Verification items for the finished model (mm, model axes). A direction names the side the tool comes from. Coordinates: 2 decimals unless noted, no trailing zeros. Write each loop counter-clockwise with the first axis right and the second up, starting at its lowest first coordinate (ties: lowest second). Pieces come first, ordered by that corner, then holes. Notation, with made-up numbers: M 36,-20 L 59,-20 A21 cw 59,0 Z; hole C 33,88 d11. An arc over 180 degrees is marked long. Answer in a Markdown table with one row per item.
from build123d import *

# Parameters (mm, degrees)
SKETCH1_W           = 56.833752097
SKETCH1_H           = 5
BOSS_EXTRUDE1_DEPTH = 80
SKETCH2_W           = 18.416876048
SKETCH2_H           = 5
SKETCH2_W_2         = 18.416876049
BOSS_EXTRUDE2_DEPTH = 5
SKETCH3_W           = 20
SKETCH3_H           = 5
BOSS_EXTRUDE3_DEPTH = 5
CUT_EXTRUDE1_DEPTH  = 5
BOSS_EXTRUDE4_DEPTH = 5
SKETCH6_R           = 2.1
CUT_EXTRUDE2_DEPTH  = 5
SKETCH8_W           = 1.93349359
SKETCH8_H           = 7.9375
CUT_EXTRUDE3_DEPTH  = 5


with BuildPart() as part:
    # Sketch1 → Boss-Extrude1 (new body)
    with BuildSketch(Plane.XY):
        with Locations((-105.747769379, -71.943096951)):
            Rectangle(SKETCH1_W, SKETCH1_H)
    extrude(amount=BOSS_EXTRUDE1_DEPTH)

    # Sketch2 → Boss-Extrude2 (add)
    with BuildSketch(Plane(origin=(0, 0, 0), x_dir=(-1, 0, 0), z_dir=(0, 0, -1))):
        with Locations((86.539331354, -71.943096951)):
            Rectangle(SKETCH2_W, SKETCH2_H)
        with Locations((124.956207403, -71.943096951)):
            Rectangle(SKETCH2_W_2, SKETCH2_H)
    extrude(amount=BOSS_EXTRUDE2_DEPTH)

    # Sketch3 → Boss-Extrude3 (add)
    with BuildSketch(Plane.XY.offset(80)):
        with Locations((-105.747769378, -71.943096951)):
            Rectangle(SKETCH3_W, SKETCH3_H)
    extrude(amount=BOSS_EXTRUDE3_DEPTH)

    # Sketch4 → Cut-Extrude1 (cut)
    with BuildSketch(Plane.XZ.offset(74.443096951)):
        Polygon((-107.847769378, 0), (-107.847769378, 5), (-110.747769378, 5), (-110.747769378, 15), (-100.747769378, 15), (-100.747769378, 5), (-103.647769378, 5), (-103.647769378, 0), align=None)
    extrude(amount=-CUT_EXTRUDE1_DEPTH, mode=Mode.SUBTRACT)

    # Sketch5 → Boss-Extrude4 (add)
    with BuildSketch(Plane.XZ.offset(74.443096951)):
        with BuildLine():
            Line((-110.077896397, 85), (-101.417642359, 85))
            ThreePointArc((-101.417642359, 85), (-105.747769378, 87.5), (-110.077896397, 85))
        make_face()
    extrude(amount=-BOSS_EXTRUDE4_DEPTH)

    # Sketch6 → Cut-Extrude2 (cut)
    with BuildSketch(Plane.XZ.offset(74.443096951)):
        with Locations((-105.747769378, 82.5)):
            Circle(SKETCH6_R)
    extrude(amount=-CUT_EXTRUDE2_DEPTH, mode=Mode.SUBTRACT)

    # Sketch8 → Cut-Extrude3 (cut)
    with BuildSketch(Plane.XZ.offset(74.443096951)):
        with BuildLine():
            Line((-123.535910404, 45.4375), (-121.602416814, 45.4375))
            Line((-121.602416814, 45.4375), (-121.602416814, 40.681678185))
            add(Edge.make_bspline(
                [(-121.602416814, 40.681678185), (-121.601990048, 40.614365441), (-121.601180152, 40.486622809), (-121.598439266, 40.304791606), (-121.592462111, 40.143061597), (-121.582649953, 40.001032923), (-121.57194051, 39.879023265), (-121.55953718, 39.776587793), (-121.545409362, 39.693656046), (-121.529735909, 39.646438596), (-121.522914611, 39.625888922)],
                knots=[0, 0, 0, 0, 0.000201942, 0.000383235, 0.000545544, 0.000687379, 0.000810317, 0.000912872, 0.000997069, 0.00106195, 0.00106195, 0.00106195, 0.00106195], degree=3))
            add(Edge.make_bspline(
                [(-121.522914611, 39.625888922), (-121.509452841, 39.587377666), (-121.482681561, 39.510790729), (-121.426995401, 39.4013048), (-121.360408578, 39.295994704), (-121.28006619, 39.19616361), (-121.189648325, 39.099739524), (-121.084644905, 39.011371702), (-120.970198973, 38.924768446), (-120.841762659, 38.843010088), (-120.697710316, 38.767120374), (-120.537215044, 38.693859228), (-120.359436668, 38.621836124), (-120.162385483, 38.55659879), (-119.948353328, 38.492219896), (-119.716163536, 38.433044528), (-119.466897465, 38.373285603), (-119.110484454, 38.302421294), (-118.652583447, 38.225640947), (-118.096617037, 38.158746344), (-117.538892715, 38.117643369), (-117.166262368, 38.112930622), (-116.980158701, 38.110576923)],
                knots=[0, 0, 0, 0, 0.000122268, 0.000243153, 0.000367543, 0.00049543, 0.00062702, 0.00076344, 0.000906544, 0.001057397, 0.001219582, 0.001394602, 0.001586524, 0.001794692, 0.002017049, 0.002256929, 0.002513405, 0.002785948, 0.003346916, 0.003905845, 0.004465364, 0.005023615, 0.005023615, 0.005023615, 0.005023615], degree=3))
            add(Edge.make_bspline(
                [(-116.980158701, 38.110576923), (-116.820057773, 38.113012249), (-116.502227103, 38.117846831), (-116.03087379, 38.147408488), (-115.569601956, 38.201435841), (-115.122201733, 38.270116147), (-114.698159331, 38.362899945), (-114.30504593, 38.466328223), (-113.950231341, 38.591770142), (-113.631201908, 38.728435362), (-113.34875012, 38.881571653), (-113.10835998, 39.053804153), (-112.902793753, 39.238379234), (-112.797305407, 39.38023024), (-112.745871341, 39.44939403)],
                knots=[0, 0, 0, 0, 0.000480322, 0.000953531, 0.00141604, 0.001873246, 0.002310797, 0.00271773, 0.003091874, 0.003438668, 0.003758203, 0.004053391, 0.004324543, 0.004582552, 0.004582552, 0.004582552, 0.004582552], degree=3))
            add(Edge.make_bspline(
                [(-112.745871341, 39.44939403), (-112.729005179, 39.477013683), (-112.692593547, 39.536640564), (-112.655395728, 39.644154214), (-112.620539489, 39.768801799), (-112.591731131, 39.913330101), (-112.572660575, 40.077680361), (-112.556459045, 40.261639349), (-112.547195392, 40.4653388), (-112.546098513, 40.607467269), (-112.545525789, 40.681678185)],
                knots=[0, 0, 0, 0, 9.6836e-05, 0.000209055, 0.000339449, 0.000485387, 0.000650461, 0.00083559, 0.001039339, 0.001261968, 0.001261968, 0.001261968, 0.001261968], degree=3))
            Line((-112.545525789, 40.681678185), (-112.545525789, 45.4375))
            Line((-112.545525789, 45.4375), (-110.612032199, 45.4375))
            Line((-110.612032199, 45.4375), (-110.612032199, 40.643517127))
            add(Edge.make_bspline(
                [(-110.612032199, 40.643517127), (-110.613477985, 40.557066925), (-110.616304371, 40.388064256), (-110.640769365, 40.140467174), (-110.679895535, 39.905487365), (-110.735004886, 39.682744005), (-110.809098914, 39.474292467), (-110.896164276, 39.27658251), (-111.0014758, 39.092896663), (-111.122090727, 38.918520772), (-111.268585123, 38.754239806), (-111.446943017, 38.599798583), (-111.654606494, 38.447346515), (-111.896614725, 38.305011699), (-112.166840551, 38.161605162), (-112.472452702, 38.030539583), (-112.807571473, 37.899478019), (-113.173034335, 37.776537822), (-113.564411059, 37.663960183), (-113.977877444, 37.566073163), (-114.411114346, 37.481431072), (-114.864742005, 37.413412032), (-115.339029089, 37.361729677), (-115.833216674, 37.323441827), (-116.347647026, 37.301283236), (-116.697109796, 37.298097825), (-116.875215793, 37.296474359)],
                knots=[0, 0, 0, 0, 0.000259299, 0.000506907, 0.000745568, 0.000973483, 0.001194247, 0.001408484, 0.001620694, 0.001828461, 0.002043564, 0.002279004, 0.00253502, 0.002815347, 0.003120457, 0.003452228, 0.003812172, 0.004199846, 0.00460849, 0.005033493, 0.005474119, 0.005932411, 0.00640914, 0.006905114, 0.007419181, 0.007953495, 0.007953495, 0.007953495, 0.007953495], degree=3))
            add(Edge.make_bspline(
                [(-116.875215793, 37.296474359), (-117.06868425, 37.298263057), (-117.448310552, 37.301772862), (-118.007268603, 37.321598277), (-118.54476417, 37.359249175), (-119.061557452, 37.406637359), (-119.556559089, 37.473190008), (-120.031185303, 37.549344646), (-120.484280367, 37.644235623), (-120.914952743, 37.748913991), (-121.317062778, 37.867570667), (-121.686773306, 37.99560829), (-122.022012304, 38.133781626), (-122.322535304, 38.280698867), (-122.589545148, 38.436491218), (-122.820107968, 38.603041936), (-123.018555474, 38.777795338), (-123.126131339, 38.907884929), (-123.178150488, 38.970790765)],
                knots=[0, 0, 0, 0, 0.000580421, 0.001138909, 0.001677586, 0.002196696, 0.002695479, 0.003175675, 0.003638446, 0.004083865, 0.004504975, 0.004895702, 0.005257132, 0.005592062, 0.005898574, 0.006183231, 0.006444425, 0.006688987, 0.006688987, 0.006688987, 0.006688987], degree=3))
            add(Edge.make_bspline(
                [(-123.178150488, 38.970790765), (-123.207601979, 39.012390462), (-123.269314795, 39.099558693), (-123.338519525, 39.254004353), (-123.400520367, 39.428804251), (-123.451403362, 39.627250965), (-123.487616881, 39.848734436), (-123.517131787, 40.092676277), (-123.531645378, 40.360316763), (-123.534449497, 40.546512034), (-123.535910404, 40.643517127)],
                knots=[0, 0, 0, 0, 0.000152586, 0.00031973, 0.000505303, 0.000708928, 0.000933214, 0.001178169, 0.001445769, 0.001736816, 0.001736816, 0.001736816, 0.001736816], degree=3))
            Line((-123.535910404, 40.643517127), (-123.535910404, 45.4375))
        make_face()
        Polygon((-104.781022583, 44.623397436), (-104.781022583, 45.4375), (-94.502977712, 45.4375), (-102.539060444, 38.314102564), (-94.910028994, 38.314102564), (-94.910028994, 37.5), (-105.595125148, 37.5), (-97.557452371, 44.623397436), align=None)
        with Locations((-88.621086686, 41.46875)):
            Rectangle(SKETCH8_W, SKETCH8_H)
    extrude(amount=-CUT_EXTRUDE3_DEPTH, mode=Mode.SUBTRACT)


solid = part.part
1) Sectioned sample at A-A (z = 8). Record the cut outline in (x, y).
Response values:
| item | result |
|---|---|
| outline | M -134.16,-74.44 L -110.75,-74.44 L -110.75,-69.44 L -134.16,-69.44 Z; M -100.75,-74.44 L -77.33,-74.44 L -77.33,-69.44 L -100.75,-69.44 Z |
2) Release check for a two-part mould opening along Z. For faces 1 (the face through (-89.588, -72, 41)), 2 (the face through (-112, -72, 0)), 3 (the face through (-95.748, -72, 82)), 4 (the face through (-123, -72, 45.438)) record: +Z half, -Z half, draft (parallel to the pull), parting line (faces both ways), or undercut.
Response values:
| item | result |
|---|---|
| face 1 | undercut |
| face 2 | -Z half |
| face 3 | draft |
| face 4 | undercut |
3) Depth check by flat-ended pin: pin 1 (1.5 mm diameter, centred on x = -88, y = -71.5, fed in from +Z); pin 2 (3 mm diameter, centred on x = -104, y = -70.5, fed in from -Z); pin 3 (3.5 mm diameter, centred on x = -105.75, z = 82.5, fed in from -Y); pin 4 (2.5 mm diameter, centred on x = -102, y = -72.5, fed in from +Z). Enter the tip coordinate at first touch or a pass-through.
Response values:
| item | result |
|---|---|
| pin 1 | stops at z = 80 |
| pin 2 | stops at z = 0 |
| pin 3 | passes through |
| pin 4 | stops at z = 86.83 |
4) Sectioned sample at B-B (x = -109). Record the cut outline in (y, z), then the cut area to 3 significant figures.
Response values:
| item | result |
|---|---|
| outline | M -74.44,0 L -69.44,0 L -69.44,5 L -74.44,5 Z; M -74.44,15 L -69.44,15 L -69.44,86.3 L -74.44,86.3 Z |
| area | 381 mm² |
5) Sectioned sample at D-D (y = -73.35). Give the number of separate pieces and of enclosed holes in the cut face, then the cut area to 3 significant figures.
Response values:
| item | result |
|---|---|
| separate pieces | 1 |
| enclosed holes | 4 |
| area | 4,630 mm² |
6) Tool access check on faces 5 (the face through (-89, -72, 45.438)), 6 (the face through (-113, -72, 85)), 7 (the face through (-95.748, -72, -2)). Record the directions out of +Z, -Z, +X, -X, +Y, -Y that give a thin tool (end or side, any length) a straight path to the whole face; none if there is none.
Response values:
| item | result |
|---|---|
| face 5 | +Y, -Y |
| face 6 | +Z, -X, +Y, -Y |
| face 7 | -Z, +Y, -Y |
7) Sectioned sample at C-C (z = 43.5). Record the cut outline in (x, y).
Response values:
| item | result |
|---|---|
| outline | M -134.16,-74.44 L -123.54,-74.44 L -123.54,-69.44 L -134.16,-69.44 Z; M -121.6,-74.44 L -112.55,-74.44 L -112.55,-69.44 L -121.6,-69.44 Z; M -110.61,-74.44 L -98.83,-74.44 L -98.83,-69.44 L -110.61,-69.44 Z; M -96.69,-74.44 L -89.59,-74.44 L -89.59,-69.44 L -96.69,-69.44 Z; M -87.65,-74.44 L -77.33,-74.44 L -77.33,-69.44 L -87.65,-69.44 Z |
8) Thickness scan on L1, parallel to Z at x = -100, y = -71.8; L2, parallel to Z at x = -122, y = -69.7; L3, parallel to Z at x = -103.5, y = -74.2. Record the ranges inside material, lowest first. Write a range as [from, to].
Response values:
| item | result |
|---|---|
| L1 | z = [0, 37.5], [38.31, 40.56], [42.46, 44.62], [45.44, 85] |
| L2 | z = [-5, 38.13], [45.44, 80] |
| L3 | z = [0, 5], [15, 37.5], [39.36, 44.62], [45.44, 86.97] |
